Could you check a few things on this model? Use its own coordinates, in mm. A direction names the side the tool comes from. Coordinates: 2 decimals unless noted, no trailing zeros. Answer as a JSON object with one key per item and string values. Group by question number.
(1) Please list where these lines run through material, in increasing order: probe 1 along Z at (x, y) = (330, 4); probe 2 along Z at (x, y) = (330, 13).
(2) We'd pull the mould along Z, two halves only. Please class faces 1 (the flat face through (-5, 7, -237.5)), 2 (the flat face through (325, 10, -139)), 3 (the flat face through (5, 7, 237.5)): pulls with the +Z half, pulls with the -Z half, needs draft (parallel to the pull), parting line crosses it, or undercut.
(3) Which directions (+Z, -Z, +X, -X, +Y, -Y) give clear straight access to the entire face, cutting with the end or side of a thin tool? Please do faces 4 (the flat face through (-325, 10, 139)), 5 (the flat face through (5, 0, 3)).
(4) Will this pin go through, and if not, where does the flat tip stop? P1, Ø13, axis at x = -330, z = -137.5, coming from the +Y side.
Autodesk Inventor part; units mm, degrees
ref_plane "YZ Plane" through (0, 0, 0) normal (1, 0, 0) x (0, 1, 0)
ref_plane "XZ Plane" through (0, 0, 0) normal (0, 1, 0) x (-1, 0, 0)
ref_plane "XY Plane" through (0, 0, 0) normal (0, 0, 1) x (1, 0, 0)
sketch "Sketch1" plane through (0, 0, 0) normal (0, 1, 0) x (-1, 0, 0)
  line L0 (345, -237.5) -> (-345, -237.5)
  line L1 (-345, -237.5) -> (-345, 237.5)
  line L2 (-345, 237.5) -> (345, 237.5)
  line L3 (345, 237.5) -> (345, -237.5)
  line L4 (345, -237.5) -> (-345, 237.5) construction
  line L5 (-345, -237.5) -> (345, 237.5) construction
  point P0 (0, 0)
  dimension "d0" = 690
  dimension "d1" = 475
extrude "Plate1" add sketch "Sketch1" along normal blind 15
sketch "Sketch2" plane through (0, 15, 0) normal (0, 1, 0) x (1, 0, 0)
  line L0 (-345, -237.5) -> (-345, 237.5) construction
  line L1 (345, -237.5) -> (-345, -237.5) construction
  line L2 (345, 237.5) -> (345, -237.5) construction
  line L3 (-345, 237.5) -> (345, 237.5) construction
  line L4 (330, -237.5) -> (330, 237.5) construction
  line L5 (345, 0) -> (0, 0) construction
  point P0 (330, -137.5)
  point P1 (330, 137.5)
  dimension "d4" = 330
  dimension "d5" = 275
  dimension "d6" = 100
  dimension "d7" = 100
hole "Hole1" at (330, 15, 137.5) at (330, 15, -137.5) direction (0, -1, 0) diameter 10 end through all counterbore diameter 14 counterbore depth 5
mirror "Mirror1" about plane through (0, 0, 0) normal (1, 0, 0) of "Hole1"
equation "\"d13\" = Thickness"
equation "\"d2\" = Thickness"
equation "\"BendRadius\" = Thickness"
equation "\"BendReliefWidth\" = Thickness"
equation "\"BendReliefDepth\" = 0.5 * Thickness"
equation "\"TransitionRadius\" = BendRadius"
equation "\"JacobiRadiusSize\" = BendRadius"
equation "\"GapSize\" = Thickness"
properties part number "фанера1" material "Wood (Maple)"
Result set:
{
 "1": {"probe 1": "z = -237.5 to -142.5, -132.5 to 132.5, 142.5 to 237.5", "probe 2": "z = -237.5 to -144.5, -130.5 to 130.5, 144.5 to 237.5"},
 "2": {"face 1": "pulls with the -Z half", "face 2": "undercut", "face 3": "pulls with the +Z half"},
 "3": {"face 4": "+Y", "face 5": "+Z, -Z, +X, -X, -Y"},
 "4": {"P1": "stops at y = 10"}
}
